from build123d import *

# Parameters (mm, degrees)
F0_R     = 3.9
F0_R_2   = 3.15
F1_DEPTH = 0.87
F2_DEPTH = 0.77
F3_DEPTH = 1.37
F4_DEPTH = 1.35
F5_R     = 0.25


with BuildPart() as f1:
    # F0 (on Top) → F1 (new body)
    with BuildSketch(Plane.XY):
        with BuildLine():
            Line((-4.75, -6.75), (6.25, -6.75))
            ThreePointArc((6.25, -6.75), (6.603553, -6.603553), (6.75, -6.25))
            Line((6.75, -6.25), (6.75, 4.75))
            ThreePointArc((6.75, 4.75), (5.335786, 5.335786), (4.75, 6.75))
            Line((4.75, 6.75), (-6.25, 6.75))
            ThreePointArc((-6.25, 6.75), (-6.603553, 6.603553), (-6.75, 6.25))
            Line((-6.75, 6.25), (-6.75, -4.75))
            ThreePointArc((-6.75, -4.75), (-5.335786, -5.335786), (-4.75, -6.75))
        make_face()
        Polygon((6.25, -6.25), (3.592141, -6.25), (6.25, -3.619419), align=None, mode=Mode.SUBTRACT)
        Polygon((-6.25, 3.592141), (-6.25, 6.25), (-3.619419, 6.25), align=None, mode=Mode.SUBTRACT)
        Circle(F0_R, mode=Mode.SUBTRACT)
        Circle(F0_R)
        Circle(F0_R_2, mode=Mode.SUBTRACT)
        Circle(F0_R_2)
    extrude(amount=F1_DEPTH)

    # F0 (on Top) → F2 (join)
    with BuildSketch(Plane.XY):
        Polygon((-3.619419, 6.25), (-6.25, 6.25), (-6.25, 3.592141), align=None)
        Polygon((6.25, -3.619419), (3.592141, -6.25), (6.25, -6.25), align=None)
    extrude(amount=F2_DEPTH)

    # F0 (on Top) → F3 (join)
    with BuildSketch(Plane.XY):
        Circle(F0_R)
        Circle(F0_R_2, mode=Mode.SUBTRACT)
    extrude(amount=F3_DEPTH)

    # F0 (on Top) → F4 (join)
    with BuildSketch(Plane.XY):
        Circle(F0_R_2)
    extrude(amount=F4_DEPTH)

    # F5
    f5_edges = [f1.edges().sort_by_distance(p)[0] for p in [
        (-3.9, 0, 1.37),
    ]]
    fillet(f5_edges, radius=F5_R)


solid = f1.part
The model under review builds one solid part; all positions refer to its coordinate system, in mm. A direction names the side the tool comes from. Round coordinates to 2 decimals unless told otherwise and drop trailing zeros. Loops run counter-clockwise (first coordinate to the right, second up) from the corner with the lowest first, then second, coordinate; pieces in that order, holes last. Notation, with made-up numbers: (44, -15.5) -> (102, -15.5) arc R30 ccw to (102, 6.5) -> close; hole circle Ø1 at (1.5, -13). An arc over 180 degrees is marked (long way). One line per question, with ' | ' between items. Start each with the question number.
Item 1: Wall thickness on line 1 along Z through (x, y) = (-4.5, -0.75); line 2 along Z through (x, y) = (-2, -0.75); line 3 along Y through (x, z) = (4, 0.8): over which ranges is each line inside the solid? List them lowest first. Write a range as [from, to].
Item 2: For pin 1 (0.8 mm diameter, centred on x = 4.5, y = -5, fed in from +Z), flat-tipped, find the tip position at first contact; note if it passes through.
Item 3: Draft analysis for pull direction X (two halves, no side actions). For faces 1 (the face through (5.35, 5.32, 0.43)), 2 (the face through (5, -6, 0.77)), 3 (the face through (-5.35, -5.32, 0.43)), state which applies: +X half, -X half, draft (parallel to the pull), parting line (faces both ways), or undercut.
Item 4: Add section D-D, the plane y = 5.25. Write out the cut boundary in (x, z).
Item 5: Machinability: for faces 4 (the face through (0, 0, 1.35)), 5 (the face through (-6.75, 0.8, 0.4)), which of the approach directions +Z, -Z, +X, -X, +Y, -Y give a long, thin tool a straight path to every point of the face, cutting with its end or side? Answer none if there is none.
Item 6: Add section B-B, the plane z = 0.55. Write out the cut boundary in (x, y).
Return value:
1) line 1: z = [0, 0.87] | line 2: z = [0, 1.35] | line 3: y = [-6.75, -6.25], [-5.85, 6.75]
2) pin 1: stops at z = 0.87
3) face 1: +X half | face 2: undercut | face 3: -X half
4) outline: (-6.75, 0) -> (5.43, 0) -> (5.43, 0.87) -> (-4.61, 0.87) -> (-4.61, 0.77) -> (-6.25, 0.77) -> (-6.25, 0.87) -> (-6.75, 0.87) -> close
5) face 4: +Z | face 5: +Z, -Z, -X, +Y, -Y
6) outline: (-6.75, -4.75) arc R2 cw to (-4.75, -6.75) -> (6.25, -6.75) arc R0.5 ccw to (6.75, -6.25) -> (6.75, 4.75) arc R2 cw to (4.75, 6.75) -> (-6.25, 6.75) arc R0.5 ccw to (-6.75, 6.25) -> close
